Here's how the part is built. I have some questions about the finished solid (model axes, mm). A direction names the side the tool comes from. Give positions to 0.01 mm unless a question says otherwise; leave off trailing zeros. Write each loop counter-clockwise with the first axis right and the second up, starting at its lowest first coordinate (ties: lowest second). Pieces come first, ordered by that corner, then holes. Notation, with made-up numbers: (-10.5, 2.25) -> (-3.5, 2.25) arc R6 ccw to (-3.5, 8.25) -> close; hole circle Ø5 at (77, 34). An arc over 180 degrees is marked (long way). Use one line per item in the form item = value.
```python
from build123d import *

# Parameters (mm, degrees)
SKETCH_1_W          = 10
SKETCH_1_H          = 20
SKETCH_1_W_2        = 7.6
SKETCH_1_H_2        = 17.6
EXTRUDE_1_DEPTH     = 350
SKETCH_2_R          = 2.15
SKETCH_2_R_2        = 6
CUT_EXTRUDE_1_DEPTH = 351.285597763
SKETCH_3_R          = 3.175
SKETCH_3_R_2        = 2.15
CUT_EXTRUDE_2_DEPTH = 351.606617165
CUT_EXTRUDE_3_REACH = 352.286
SKETCH_4_W          = 99
SKETCH_4_H          = 20


with BuildPart() as part:
    # ｽｹｯﾁ1 → 押し出し-薄板1 (new body)
    with BuildSketch(Plane(origin=(0, 0, 0), x_dir=(0, 0, -1), z_dir=(1, 0, 0))):
        Rectangle(SKETCH_1_W, SKETCH_1_H)
        Rectangle(SKETCH_1_W_2, SKETCH_1_H_2, mode=Mode.SUBTRACT)
    extrude(amount=EXTRUDE_1_DEPTH)

    # ｽｹｯﾁ2 → ｶｯﾄ - 押し出し1 (cut, through all)
    with BuildSketch(Plane.XY.offset(5)):
        with Locations((246, 5)):
            Circle(SKETCH_2_R)
        with Locations(Location((246, -5, 0), (0, 0, 90))):
            Circle(SKETCH_2_R)
        with Locations((5, -5)):
            Circle(SKETCH_2_R)
        with Locations(Location((5, 5, 0), (0, 0, 90))):
            Circle(SKETCH_2_R)
        with Locations((164.5, 0)):
            Circle(SKETCH_2_R)
        with Locations((144.5, 0)):
            Circle(SKETCH_2_R)
        with Locations((124.5, 0)):
            Circle(SKETCH_2_R)
        with Locations((330, 0)):
            Circle(SKETCH_2_R_2)
        with Locations((308, 0)):
            Circle(SKETCH_2_R_2)
        with Locations((286, 0)):
            Circle(SKETCH_2_R_2)
        with Locations((264, 0)):
            Circle(SKETCH_2_R_2)
        with Locations((228, 0)):
            Circle(SKETCH_2_R_2)
        with Locations((206, 0)):
            Circle(SKETCH_2_R_2)
        with Locations((184, 0)):
            Circle(SKETCH_2_R_2)
        with Locations((106.5, 0)):
            Circle(SKETCH_2_R_2)
        with Locations((84.5, 0)):
            Circle(SKETCH_2_R_2)
        with Locations((62.5, 0)):
            Circle(SKETCH_2_R_2)
        with Locations((40.5, 0)):
            Circle(SKETCH_2_R_2)
        with Locations((18.5, 0)):
            Circle(SKETCH_2_R_2)
    extrude(amount=-CUT_EXTRUDE_1_DEPTH, mode=Mode.SUBTRACT)

    # ｽｹｯﾁ3 → ｶｯﾄ - 押し出し2 (cut, through all)
    with BuildSketch(Plane(origin=(0, 10, 0), x_dir=(1, 0, 0), z_dir=(0, 1, 0))):
        with Locations(Location((343.25, 0, 0), (0, 0, 270))):
            Circle(SKETCH_3_R)
        with Locations(Location((173.7, 0, 0), (0, 0, 270))):
            Circle(SKETCH_3_R_2)
        with Locations(Location((203.7, 0, 0), (0, 0, 270))):
            Circle(SKETCH_3_R_2)
    extrude(amount=-CUT_EXTRUDE_2_DEPTH, mode=Mode.SUBTRACT)

    # ｶｯﾄ - 押し出し3: up to this face of the body (flat: up to its plane)
    cut_extrude_3_end = Plane(part.part.faces().sort_by_distance((175.381114236, 0, -5))[0])
    # ｽｹｯﾁ4 → ｶｯﾄ - 押し出し3 (cut, up to the picked face)
    with BuildSketch(Plane.XY.offset(5), mode=Mode.PRIVATE) as cut_extrude_3_sk1:
        with Locations((300.5, 0)):
            Rectangle(SKETCH_4_W, SKETCH_4_H)
    cut_extrude_3_tool1 = split(extrude(cut_extrude_3_sk1.sketch, amount=-CUT_EXTRUDE_3_REACH, mode=Mode.PRIVATE), bisect_by=cut_extrude_3_end, keep=Keep.BOTH, mode=Mode.PRIVATE)
    add(cut_extrude_3_tool1.solids().sort_by(Axis((300.5, 0, 5), (0, 0, -1)))[0], mode=Mode.SUBTRACT)


solid = part.part
```
Q1. I want a section at A-A, the plane x = 40.5. Write out the boundary of the cut face in (y, z).
Result set:
outline = (-10, -5) -> (-6, -5) -> (-6, -3.8) -> (-8.8, -3.8) -> (-8.8, 3.8) -> (-6, 3.8) -> (-6, 5) -> (-10, 5) -> close; (6, -5) -> (10, -5) -> (10, 5) -> (6, 5) -> (6, 3.8) -> (8.8, 3.8) -> (8.8, -3.8) -> (6, -3.8) -> close
Q2. I want a section at B-B, the plane x = 246. Write out the boundary of the cut face in (y, z).
Result set:
outline = (-10, -5) -> (-7.15, -5) -> (-7.15, -3.8) -> (-8.8, -3.8) -> (-8.8, 3.8) -> (-7.15, 3.8) -> (-7.15, 5) -> (-10, 5) -> close; (-2.85, -5) -> (2.85, -5) -> (2.85, -3.8) -> (-2.85, -3.8) -> close; (-2.85, 3.8) -> (2.85, 3.8) -> (2.85, 5) -> (-2.85, 5) -> close; (7.15, -5) -> (10, -5) -> (10, 5) -> (7.15, 5) -> (7.15, 3.8) -> (8.8, 3.8) -> (8.8, -3.8) -> (7.15, -3.8) -> close
Q3. If I drill on line 1 along Z through (x, y) = (142.5, 3.5); line 2 along Y through (x, z) = (84, 3); line 3 along Z through (x, y) = (203.7, 9.25), over which ranges is the centre line in solid material (lowest first)? Write a range as from..to.
Result set:
line_1 = -5..-3.8, 3.8..5
line_2 = -10..-8.8, 8.8..10
line_3 = -5..-2.15, 2.15..5
Q4. If we mould it in two halves opening along X, with no side actions, what happens to faces 1 (the face through (166.486, -0.823, -4.392)), 2 (the face through (175.51, -9.39, 1.16)), 3 (the face through (251, 0, 4)), 4 (the face through (124, 10, 0))? For each: +X half, -X half, draft (parallel to the pull), parting line (faces both ways), or undercut.
Result set:
face_1 = undercut
face_2 = undercut
face_3 = +X half
face_4 = draft
Q5. I want a section at C-C, the plane z = 0.5. Write out the boundary of the cut face in (x, y), and give its area (3 significant figures).
Result set:
outline = (0, -10) -> (171.61, -10) -> (171.61, -8.8) -> (0, -8.8) -> close; (0, 8.8) -> (171.61, 8.8) -> (171.61, 10) -> (0, 10) -> close; (175.79, -10) -> (201.61, -10) -> (201.61, -8.8) -> (175.79, -8.8) -> close; (175.79, 8.8) -> (201.61, 8.8) -> (201.61, 10) -> (175.79, 10) -> close; (205.79, -10) -> (251, -10) -> (251, -8.8) -> (205.79, -8.8) -> close; (205.79, 8.8) -> (251, 8.8) -> (251, 10) -> (205.79, 10) -> close
area = 582 mm2
Q6. Which directions (+Z, -Z, +X, -X, +Y, -Y) give clear straight access to the entire face, cutting with the end or side of a thin tool? Please do faces 5 (the face through (201.24, -3.65, 4.41)), 6 (the face through (124, -4, 3.8)).
Result set:
face_5 = +Z, -Z
face_6 = +X, -X
Q7. I want a section at D-D, the plane x = 124.5. Write out the boundary of the cut face in (y, z), and give its area (3 significant figures).
Result set:
outline = (-10, -5) -> (-2.15, -5) -> (-2.15, -3.8) -> (-8.8, -3.8) -> (-8.8, 3.8) -> (-2.15, 3.8) -> (-2.15, 5) -> (-10, 5) -> close; (2.15, -5) -> (10, -5) -> (10, 5) -> (2.15, 5) -> (2.15, 3.8) -> (8.8, 3.8) -> (8.8, -3.8) -> (2.15, -3.8) -> close
area = 55.9 mm2
